Autodesk Inventor part; units mm, degrees
ref_plane "YZ Plane" through (0, 0, 0) normal (1, 0, 0) x (0, 1, 0)
ref_plane "XZ Plane" through (0, 0, 0) normal (0, 1, 0) x (-1, 0, 0)
ref_plane "XY Plane" through (0, 0, 0) normal (0, 0, 1) x (1, 0, 0)
sketch "スケッチ1" plane through (0, 0, 0) normal (0, 0, 1) x (1, 0, 0)
  line L0 (-22.5, 3.5) -> (22.5, 3.5)
  line L1 (22.5, 3.5) -> (22.5, -3.5)
  line L2 (22.5, -3.5) -> (-22.5, -3.5)
  line L3 (-22.5, -3.5) -> (-22.5, 3.5)
  line L4 (-22.5, 3.5) -> (22.5, -3.5) construction
  line L5 (22.5, 3.5) -> (-22.5, -3.5) construction
  line L6 (0, -6.37) -> (0, 6.37) construction
  line L7 (-34.37, 0) -> (34.37, 0) construction
  circle A0 centre (-20, 0) radius 4.55
  line L8 (22.5, -3.5) -> (22.5, 3.5)
  circle A1 centre (20, 0) radius 4.55
  circle A2 centre (-20, 0) radius 1.635
  circle A3 centre (20, 0) radius 1.635
  line L9 (14, 3.5) -> (14, -3.5)
  line L10 (16, 3.5) -> (16, -3.5)
  point P0 (0, 0)
  point P1 (-17.0927, 3.5)
  point P2 (-22.9073, 3.5)
  point P3 (-22.9073, -3.5)
  point P4 (-17.0927, -3.5)
  point P5 (17.0927, 3.5)
  point P6 (17.0927, -3.5)
  point P7 (22.9073, -3.5)
  point P8 (22.9073, 3.5)
  dimension "d1" = 7
  dimension "d2" = 20
  dimension "d3" = 45
  dimension "d4" = 9.1
  dimension "d12" = 3.27
  dimension "d13" = 3.27
  dimension "d14" = 6
  dimension "d15" = 2
extrude "押し出し1" add sketch "スケッチ1" along normal mid plane 5 contours L9 L2 A0 L0 | L0 L10 A1 L2 L9 | L0 A1 L10 | A0 L2 L3 L0 | L0 L1 L2 A1 L10 | L10 A1 | L10 A1 L2 picked at (-19.7985, 2.8744)
fillet "フィレット1" radius 3 4 edges at (-22.5, 3.5, 0) (-22.5, -3.5, 0) (22.5, -3.5, 0) (22.5, 3.5, 0)
properties part number "link_arm_1"
Part model, mm, in its own coordinate system. Round coordinates to 2 decimals unless told otherwise and drop trailing zeros. Loops run counter-clockwise (first coordinate to the right, second up) from the corner with the lowest first, then second, coordinate; pieces in that order, holes last. Notation, with made-up numbers: (-24, -19.5) -> (30, -19.5) arc R21 cw to (30, 8.5) -> close; hole circle Ø3 at (68, 25). An arc over 180 degrees is marked (long way). Use CSV: the item, a comma, the result in double quotes. Start each with the question number.
1) Cut at D-D, the plane y = 2.25. Write the cut outline in (x, z).
2) Cut at A-A, the plane y = 0. Write the cut outline in (x, z) (3 decimals).
3) Cut at B-B, the plane x = -20. Write the cut outline in (y, z) (3 decimals), plus the area to 3 significant figures.
4) Wall check: L1, parallel to X at y = 0.75, z = -2.2; L2, parallel to X at y = -0.25, z = 1.25; L3, parallel to Y at x = -20, z = 1.45 (3 decimals). Give the ranges that are in metal, low to high. Write a range as [from, to].
5) Pull direction X, two halves, no side cores. Call faces 1 (the cylindrical face through (21.64, 2.6, 0.04)), 2 (the cylindrical face through (21.51, 0.63, -0.04)), 3 (the cylindrical face through (-21.6, -2.64, -0.04)): +X half, -X half, draft (parallel to the pull), parting line (faces both ways), or undercut.
6) Cut at C-C, the plane z = 0.7. Write the cut outline in (x, y) (3 decimals), plus the area to 3 significant figures.
Determined:
1,outline,"(-21.94, -2.5) -> (21.94, -2.5) -> (21.94, 2.5) -> (-21.94, 2.5) -> close"
2,outline,"(-22.5, -2.5) -> (-21.635, -2.5) -> (-21.635, 2.5) -> (-22.5, 2.5) -> close; (-18.365, -2.5) -> (18.365, -2.5) -> (18.365, 2.5) -> (-18.365, 2.5) -> close; (21.635, -2.5) -> (22.5, -2.5) -> (22.5, 2.5) -> (21.635, 2.5) -> close"
3,outline,"(-3.458, -2.5) -> (-1.635, -2.5) -> (-1.635, 2.5) -> (-3.458, 2.5) -> close; (1.635, -2.5) -> (3.458, -2.5) -> (3.458, 2.5) -> (1.635, 2.5) -> close"
3,area,"18.2 mm2"
4,L1,"x = [-22.49, -21.45], [-18.55, 18.55], [21.45, 22.49]"
4,L2,"x = [-22.5, -21.62], [-18.38, 18.38], [21.62, 22.5]"
4,L3,"y = [-3.458, -1.635], [1.635, 3.458]"
5,face 1,"+X half"
5,face 2,"undercut"
5,face 3,"-X half"
6,outline,"(-22.5, -0.5) arc R3 ccw to (-19.5, -3.5) -> (19.5, -3.5) arc R3 ccw to (22.5, -0.5) -> (22.5, 0.5) arc R3 ccw to (19.5, 3.5) -> (-19.5, 3.5) arc R3 ccw to (-22.5, 0.5) -> close; hole circle Ø3.27 at (-20, 0); hole circle Ø3.27 at (20, 0)"
6,area,"290 mm2"
